Source: CAD feature listing. Evaluate the final solid. Frame: model axes, mm. Face numbers are marked on the shaded views. A direction names the side the tool comes from. Coordinates: 2 decimals unless noted, no trailing zeros. Loops run counter-clockwise (first coordinate to the right, second up) from the corner with the lowest first, then second, coordinate; pieces in that order, holes last.
Item 1: Line query: probe 1 along Y at (x, z) = (0, 7.75); probe 2 along X at (y, z) = (1.45, 20); probe 3 along Y at (x, z) = (0, 4). Output: solid intervals per line, ascending.
Item 2: Section query C-C, the plane x = 15. Return the cut outline in (y, z).
Item 3: Section query D-D, the plane x = -20. Return the cut outline in (y, z), then the cut area to 3 significant figures.
Item 4: Section query A-A, the plane z = 8.5. State how many separate pieces and enclosed holes the cut face has, then the cut area to 3 significant figures.
Item 5: Pin query (flat end, axial travel): pin 1 Ø9 at (y, z) = (22.5, 8) entering from +X; pin 2 Ø8 at (x, y) = (-15, 19.5) entering from -Z; pin 3 Ø4 at (y, z) = (25, 6) entering from -X; pin 4 Ø21 at (x, y) = (-0.5, 31) entering from +Z. Return the tip coordinate at first contact, or that it passes through.
Item 6: Pull-direction query (Y, two-part tool) for the marked faces 1, 2, 3 and 4; classes: +Y half, -Y half, draft (parallel to the pull), parting line (faces both ways), or undercut.
Item 7: Reachability of the marked faces 5, 6 and 7 from +Z, -Z, +X, -X, +Y, -Y: full face, straight path, thin tool, end or side. Return the list, or none.
Item 8: Section query B-B, the plane z = 20. Return the cut outline in (x, y).
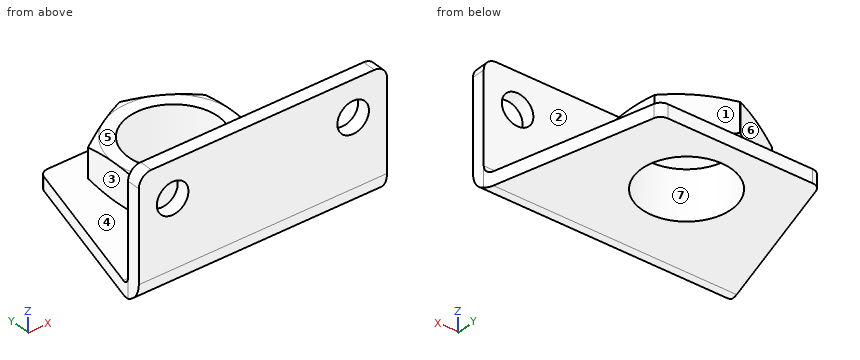
```python
from build123d import *

# Parameters (mm, degrees)
EXTRUDE_START            = 27.5
EXTRUDE_1_DEPTH          = 55
EXTRUDE_2_DEPTH          = 8
CUT_EXTRUDE_1_DEPTH      = 55.608961566
CUT_EXTRUDE_1_DEPTH_BACK = 55.608961566
SKETCH_4_R               = 10
CUT_EXTRUDE_2_DEPTH      = 55.608961566
CUT_EXTRUDE_2_DEPTH_BACK = 55.608961566
SKETCH_6_R               = 3.5
CUT_EXTRUDE_3_DEPTH      = 54.937463789
FILLET_1_R               = 2
FILLET_2_R               = 2.8


with BuildPart() as part:
    # 草图3 → 凸台-拉伸1 (new body)
    with BuildSketch(Plane(origin=(0, 0, 0), x_dir=(0, 0, -1), z_dir=(1, 0, 0)).offset(EXTRUDE_START)):
        with BuildLine():
            Line((-28, 0), (-5, 0))
            ThreePointArc((-5, 0), (-1.464466094, 1.464466094), (0, 5))
            Line((0, 5), (0, 40))
            Line((0, 40), (-3, 40))
            Line((-3, 40), (-3, 5))
            ThreePointArc((-3, 5), (-3.585786438, 3.585786438), (-5, 3))
            Line((-5, 3), (-28, 3))
            Line((-28, 3), (-28, 0))
        make_face()
    extrude(amount=-EXTRUDE_1_DEPTH)

    # 草图7 → 凸台-拉伸2 (add)
    with BuildSketch(Plane.XY.offset(3)):
        Polygon((0, 40.011106999), (-13, 32.505553499), (-13, 17.494446501), (0, 9.988893001), (13, 17.494446501), (13, 32.505553499), align=None)
    extrude(amount=EXTRUDE_2_DEPTH)

    # 草图4 → 切除-拉伸1 (cut, two sides: drawn at the far end of the back side and taken through both)
    with BuildSketch(Plane.XY.offset(3).offset(-CUT_EXTRUDE_1_DEPTH_BACK)):
        with Locations((0, 25)):
            Circle(SKETCH_4_R)
    extrude(amount=CUT_EXTRUDE_1_DEPTH + CUT_EXTRUDE_1_DEPTH_BACK, mode=Mode.SUBTRACT)

    # 草图8 → 切除-旋转1 (revolve, cut)
    with BuildSketch(Plane(origin=(0, 25, 0), x_dir=(-1, 0, 0), z_dir=(0, 1, 0))):
        Polygon((-13, 11), (-18, 11), (-18, 9.180148829), align=None)
        Polygon((-18, 3), (-18, 4.819851171), (-13, 3), align=None)
    revolve(axis=Axis((0, 25, 0), (0, 0, 1)), mode=Mode.SUBTRACT)

    # 草图5 → 切除-拉伸2 (cut, two sides: drawn at the far end of the back side and taken through both)
    with BuildSketch(Plane.XY.offset(3).offset(-CUT_EXTRUDE_2_DEPTH_BACK)):
        Polygon((-17.58587988, 40), (-27.5, 3), (-27.5, 50), (27.5, 50), (27.5, 3), (17.58587988, 40), align=None)
    extrude(amount=CUT_EXTRUDE_2_DEPTH + CUT_EXTRUDE_2_DEPTH_BACK, mode=Mode.SUBTRACT)

    # 草图6 → 切除-拉伸3 (cut, through all)
    with BuildSketch(Plane(origin=(0, 3, 0), x_dir=(1, 0, 0), z_dir=(0, 1, 0))):
        with Locations(Location((-20, -20, 0), (0, 0, 270))):
            Circle(SKETCH_6_R)
        with Locations(Location((20, -20, 0), (0, 0, 90))):
            Circle(SKETCH_6_R)
    extrude(amount=-CUT_EXTRUDE_3_DEPTH, mode=Mode.SUBTRACT)

    # 圆角1
    fillet_1_edges = [part.edges().sort_by_distance(p)[0] for p in [
        (17.58587988, 40, 1.5),
        (-17.58587988, 40, 1.5),
    ]]
    fillet(fillet_1_edges, radius=FILLET_1_R)

    # 圆角2
    fillet_2_edges = [part.edges().sort_by_distance(p)[0] for p in [
        (27.5, 1.5, 28),
        (-27.5, 1.5, 28),
    ]]
    fillet(fillet_2_edges, radius=FILLET_2_R)


solid = part.part
```
Verdict:
1. probe 1: y = 0 to 3, 9.99 to 15, 35 to 40
1. probe 2: x = -27.5 to -23.5, -16.5 to 16.5, 23.5 to 27.5
1. probe 3: y = 0.1 to 3.27, 9.99 to 15, 35 to 40
2. outline: (0, 5) arc R5 ccw to (5, 0) - (40, 0) - (40, 3) - (5, 3) arc R2 cw to (3, 5) - (3, 28) - (0, 28) - close
3. outline: (0, 5) arc R5 ccw to (5, 0) - (30.99, 0) - (30.99, 3) - (5, 3) arc R2 cw to (3, 5) - (3, 16.5) - (0, 16.5) - close; (0, 23.5) - (3, 23.5) - (3, 28) - (0, 28) - close
3. area: 142 mm2
4. separate pieces: 2
4. enclosed holes: 1
4. area: 436 mm2
5. pin 1: stops at x = 13
5. pin 2: stops at z = 0
5. pin 3: stops at x = -13
5. pin 4: stops at z = 11
6. face 1: +Y half
6. face 2: undercut
6. face 3: draft
6. face 4: undercut
7. face 5: +Z, +X, -X, +Y
7. face 6: +Z, -X, +Y
7. face 7: +Z, -Z
8. outline: (-27.5, 0) - (-23.5, 0) - (-23.5, 3) - (-27.5, 3) - close; (-16.5, 0) - (16.5, 0) - (16.5, 3) - (-16.5, 3) - close; (23.5, 0) - (27.5, 0) - (27.5, 3) - (23.5, 3) - close
